The model under review builds one solid part; all positions refer to its coordinate system, in mm. Face numbers are marked on the shaded views. A direction names the side the tool comes from. Coordinates: 2 decimals unless noted, no trailing zeros. Order: outer loops, then holes, each group sorted by start corner. A loop starts at its lowest first (then second) coordinate and runs counter-clockwise, first axis right, second up. Notation, with made-up numbers: (86, -19.5) -> (112, -19.5) arc R21 ccw to (112, 6.5) -> close; hole circle Ø2 at (-5, 26.25). An arc over 180 degrees is marked (long way). Put each result on its own line as item: value.
from build123d import *

# Parameters (mm, degrees)
SKETCH_W        = 15.5
SKETCH_H        = 10
PAD_DEPTH       = 10
POCKET_DEPTH    = 9
POCKET001_DEPTH = 10
POCKET002_DEPTH = 8.6
SKETCH002_R     = 3
HOLE_DEPTH      = 25
SKETCH012_W     = 3.2
SKETCH012_H     = 0.6
POCKET004_DEPTH = 10


with BuildPart() as part:
    # Sketch → Pad (new body)
    with BuildSketch(Plane.YZ):
        with Locations((7.75, 5)):
            Rectangle(SKETCH_W, SKETCH_H)
    extrude(amount=PAD_DEPTH)

    # Sketch001 (on Face1 of Pad) → Pocket (cut)
    with BuildSketch(Plane(origin=(0, 0, 0), x_dir=(0, 0, -1), z_dir=(0, -1, 0))):
        Polygon((-2, 6.1), (-2, 3.9), (0, 3.9), (0, 5), (0, 6.1), align=None)
    extrude(amount=-POCKET_DEPTH, mode=Mode.SUBTRACT)

    # Sketch003 → Pocket001 (cut)
    with BuildSketch(Plane.YZ.offset(10)):
        Polygon((2.15, 10), (9, 7.9), (15.5, 7.9), (15.5, 10), align=None)
    extrude(amount=-POCKET001_DEPTH, mode=Mode.SUBTRACT)

    # Sketch004 (on Face4 of Pad) → Pocket002 (cut)
    with BuildSketch(Plane(origin=(0, 0, 10), x_dir=(0, -1, 0), z_dir=(0, 0, 1))):
        Polygon((-15.5, 8.6), (-15.5, 5), (-15.5, 1.4), (-2.15, 1.4), (-2.15, 8.6), align=None)
    extrude(amount=-POCKET002_DEPTH, mode=Mode.SUBTRACT)

    # Sketch002 (on Face1 of Pocket) → Hole (cut)
    with BuildSketch(Plane(origin=(0, 0, 0), x_dir=(0, 0, -1), z_dir=(0, -1, 0))):
        with Locations((-5.5, 5)):
            Circle(SKETCH002_R)
    extrude(amount=-HOLE_DEPTH, mode=Mode.SUBTRACT)

    # Sketch012 (on Face2 of Hole) → Pocket004 (cut)
    with BuildSketch(Plane(origin=(0, 0, 0), x_dir=(0, 1, 0), z_dir=(-1, 0, 0))):
        with Locations((13.9, -5.2)):
            Rectangle(SKETCH012_W, SKETCH012_H)
    extrude(amount=-POCKET004_DEPTH, mode=Mode.SUBTRACT)


solid = part.part
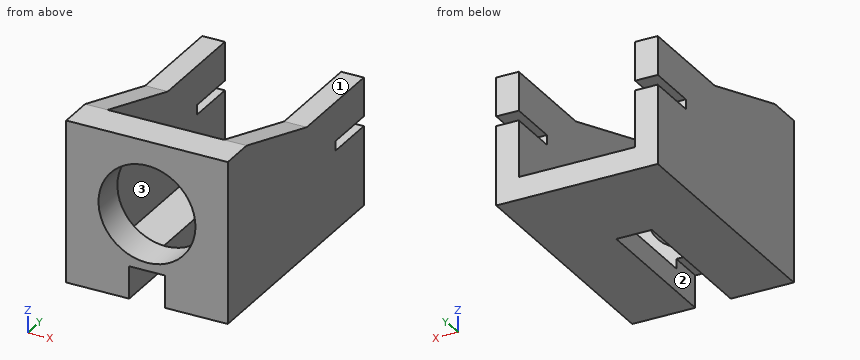
Item 1: For line 1 (X direction, y = 1.5, z = 5.5); line 2 (X direction, y = 8, z = 2); line 3 (Y direction, x = 5.5, z = 9), list the stretches that pass through material, from the lowest coordinate up. Write a range as from..to.
Answers below:
line 1: 0..2, 8..10
line 2: 0..1.4, 8.6..10
line 3: 0..2.15
Item 2: Consider section B-B on z = 3.25. Write out the cut boundary in (x, y), and give its area (3 significant figures).
Answers below:
outline: (0, 0) -> (3.02, 0) -> (3.02, 2.15) -> (1.4, 2.15) -> (1.4, 15.5) -> (0, 15.5) -> close; (6.98, 0) -> (10, 0) -> (10, 15.5) -> (8.6, 15.5) -> (8.6, 2.15) -> (6.98, 2.15) -> close
area: 50.3 mm^2
Item 3: Consider section C-C on y = 6.75. Write out the cut boundary in (x, z).
Answers below:
outline: (0, 0) -> (3.9, 0) -> (3.9, 1.4) -> (1.4, 1.4) -> (1.4, 8.59) -> (0, 8.59) -> close; (6.1, 0) -> (10, 0) -> (10, 8.59) -> (8.6, 8.59) -> (8.6, 1.4) -> (6.1, 1.4) -> close
Item 4: For the marked faces 1, 2 and 3, list the 3-axis set-ups (+Z, -Z, +X, -X, +Y, -Y) from which the entire face can be reached by the end or side of a thin tool; tool diameter is ignored.
Answers below:
face 1: +Z, +X, -X, +Y
face 2: -Z, -Y
face 3: +Z, +Y
Item 5: Consider section A-A on x = 5. Write out the cut boundary in (y, z).
Answers below:
outline: (0, 2) -> (2.15, 2) -> (2.15, 2.5) -> (0, 2.5) -> close; (0, 8.5) -> (2.15, 8.5) -> (2.15, 10) -> (0, 10) -> close; (9, 0) -> (15.5, 0) -> (15.5, 1.4) -> (9, 1.4) -> close
Item 6: Consider section D-D on y = 10. Write out the cut boundary in (x, z), and give its area (3 significant figures).
Answers below:
outline: (0, 0) -> (10, 0) -> (10, 7.9) -> (8.6, 7.9) -> (8.6, 1.4) -> (1.4, 1.4) -> (1.4, 7.9) -> (0, 7.9) -> close
area: 32.2 mm^2
Item 7: For pin 1 Ø1.1 at (x, y) = (9, 14.5) entering from +Z; pin 2 Ø1.1 at (x, y) = (5, 1.5) entering from -Z; pin 3 Ø3.5 at (x, z) = (4, 3.5) entering from +Y, all flat-tipped, find the tip position at first contact; note any pin that passes through.
Answers below:
pin 1: z = 7.9
pin 2: z = 2
pin 3: y = 2.15
